```python
from build123d import *

# Parameters (mm, degrees)
SKETCH2_R          = 1
CUT_EXTRUDE1_DEPTH = 22.53050162
CIRPATTERN1_COUNT  = 4
SKETCH5_R          = 1.25
CUT_EXTRUDE4_DEPTH = 10
SKETCH3_R          = 2.75
CUT_EXTRUDE2_DEPTH = 8
SKETCH4_R          = 2.25
CUT_EXTRUDE3_DEPTH = 2


with BuildPart() as part:
    # Sketch1 → Revolve1 (revolve)
    with BuildSketch(Plane.XY, mode=Mode.PRIVATE) as revolve1_sk:
        Polygon((0, 13.25), (0, 0), (7.5, 0), (7.5, 5.25), (8.5, 5.25), (8.5, 7.25), (12, 7.25), (12, 13.25), align=None)
    revolve(revolve1_sk.sketch.rotate(Axis((0, 0, 0), (0, 1, 0)), 90), axis=Axis((0, 0, 0), (0, 1, 0)))

    # Sketch2 → Cut-Extrude1 (cut, through all)
    with BuildSketch(Plane(origin=(0, 13.25, 0), x_dir=(1, 0, 0), z_dir=(0, 1, 0))):
        with Locations(Location((4.5, 0, 0), (0, 0, 270))):
            Circle(SKETCH2_R)
    cut_extrude1 = extrude(amount=-CUT_EXTRUDE1_DEPTH, mode=Mode.SUBTRACT)

    # CirPattern1: Cut-Extrude1 ×4 about axis
    cirpattern1_axis = Axis((0, 0, 0), (0, 1, 0))
    for i in range(1, CIRPATTERN1_COUNT):
        add(cut_extrude1.rotate(cirpattern1_axis, i * 360 / CIRPATTERN1_COUNT), mode=Mode.SUBTRACT)

    # Sketch5 → Cut-Extrude4 (cut)
    with BuildSketch(Plane(origin=(0, 13.25, 0), x_dir=(1, 0, 0), z_dir=(0, 1, 0))):
        with Locations(Location((0, 8.5, 0), (0, 0, 270))):
            Circle(SKETCH5_R)
        with Locations(Location((0, -8.5, 0), (0, 0, 270))):
            Circle(SKETCH5_R)
    extrude(amount=-CUT_EXTRUDE4_DEPTH, mode=Mode.SUBTRACT)

    # Sketch3 → Cut-Extrude2 (cut)
    with BuildSketch(Plane.XZ):
        with Locations(Location((0, 8.5, 0), (0, 0, 270))):
            Circle(SKETCH3_R)
        with Locations(Location((0, -8.5, 0), (0, 0, 270))):
            Circle(SKETCH3_R)
    extrude(amount=-CUT_EXTRUDE2_DEPTH, mode=Mode.SUBTRACT)

    # Sketch4 → Cut-Extrude3 (cut)
    with BuildSketch(Plane(origin=(0, 13.25, 0), x_dir=(1, 0, 0), z_dir=(0, 1, 0))):
        with Locations(Location((0, 0, 0), (0, 0, 270))):
            Circle(SKETCH4_R)
    extrude(amount=-CUT_EXTRUDE3_DEPTH, mode=Mode.SUBTRACT)


solid = part.part
```
Input: part model. Units: mm. Frame: model coordinates. A direction names the side the tool comes from. Coordinates: 2 decimals unless noted, no trailing zeros. Loops run counter-clockwise (first coordinate to the right, second up) from the corner with the lowest first, then second, coordinate; pieces in that order, holes last. Notation, with made-up numbers: M -16,71 L -11,71 A8 cw -11,78 Z; hole C -29.75,1.5 d8. An arc over 180 degrees is marked long. Use a Markdown table: item, result. Add a question column.
1) Section B-B, the plane y = 3. Return the cut outline in (x, z), plus the area to 3 significant figures.
2) Draft query along Z for faces 1 (the cylindrical face through (-8.5, 6.3, -0.1)), 2 (the flat face through (0, 11.25, 0)), 3 (the flat face through (7.94, 7.25, 3.5)). Return one class per face: +Z half, -Z half, draft (parallel to the pull), parting line (faces both ways), or undercut.
3) Set-up query: faces 4 (the cylindrical face through (0.121, 4.833, -5.753)), 5 (the flat face through (-8, 5.25, 0)), 6 (the cylindrical face through (7.5, 2.7, 0.1)). Return all of +Z, -Z, +X, -X, +Y, -Y with unobstructed straight access to the full face (end or side cutting, diameter ignored); none if empty.
4) Pin query (flat end, axial travel): P1, Ø3, axis at x = 0, z = 8.5, coming from the +Y side; P2, Ø1.6, axis at x = -1, z = -10, coming from the -Y side; P3, Ø5, axis at x = 8, y = 2, coming from the +Z side; P4, Ø1.2, axis at x = 0, z = -4.5, coming from the -Y side. Return the tip coordinate at first contact, or that it passes through.
5) Section D-D, the plane y = 12.25. Return the cut outline in (x, z).
6) Section A-A, the plane z = 0. Return the cut outline in (x, y), plus the area to 3 significant figures.
7) Section C-C, the plane x = 0. Give the number of separate pieces and of enclosed holes in the cut face, plus the area to 3 significant figures.
8) Line query: L1, parallel to Z at x = 0, y = 4.75; L2, parallel to X at y = 7, z = 0; L3, parallel to X at y = 7.5, z = 0. Output: solid intervals per line, ascending. Write a range as from..to.
Answer below:
| question | item | result |
|---|---|---|
| 1 | outline | M -2.38,-7.11 A2.75 cw 2.38,-7.11 A7.5 ccw 2.38,7.11 A2.75 cw -2.38,7.11 A7.5 ccw Z; hole C -4.5,0 d2; hole C 0,-4.5 d2; hole C 0,4.5 d2; hole C 4.5,0 d2 |
| 1 | area | 153 mm2 |
| 2 | face 1 | parting line |
| 2 | face 2 | undercut |
| 2 | face 3 | draft |
| 3 | face 4 | -Y |
| 3 | face 5 | -X, -Y |
| 3 | face 6 | +X, -Y |
| 4 | P1 | y = 13.25 |
| 4 | P2 | y = 8 |
| 4 | P3 | z = 5.1 |
| 4 | P4 | through |
| 5 | outline | C 0,0 d24; hole C -4.5,0 d2; hole C 0,0 d4.5; hole C 0,-8.5 d2.5; hole C 0,8.5 d2.5; hole C 0,-4.5 d2; hole C 0,4.5 d2; hole C 4.5,0 d2 |
| 6 | outline | M -12,7.25 L -8.5,7.25 L -8.5,5.25 L -7.5,5.25 L -7.5,0 L -5.5,0 L -5.5,13.25 L -12,13.25 Z; M -3.5,0 L 3.5,0 L 3.5,13.25 L 2.25,13.25 L 2.25,11.25 L -2.25,11.25 L -2.25,13.25 L -3.5,13.25 Z; M 5.5,0 L 7.5,0 L 7.5,5.25 L 8.5,5.25 L 8.5,7.25 L 12,7.25 L 12,13.25 L 5.5,13.25 Z |
| 6 | area | 195 mm2 |
| 7 | separate pieces | 5 |
| 7 | enclosed holes | 0 |
| 7 | area | 131 mm2 |
| 8 | L1 | -5.75..-5.5, -3.5..3.5, 5.5..5.75 |
| 8 | L2 | -8.5..-5.5, -3.5..3.5, 5.5..8.5 |
| 8 | L3 | -12..-5.5, -3.5..3.5, 5.5..12 |
